Geometry: final body of the model. Coordinates: model frame, mm. Face numbers are marked on the shaded views. A direction names the side the tool comes from. Give positions to 0.01 mm unless a question says otherwise; leave off trailing zeros. Write each loop counter-clockwise with the first axis right and the second up, starting at its lowest first coordinate (ties: lowest second). Pieces come first, ordered by that corner, then holes.
Q1. Section B-B (x = 10). Return the cut outline in (y, z).
Q2. Section D-D (z = -4.25). Return the cut outline in (x, y).
Q3. Section C-C (x = -4). Return the cut outline in (y, z), plus the area to 3 significant figures.
Q4. Line query: line 1 (X direction, y = 8, z = -7); line 2 (X direction, y = 15.5, z = -4); line 3 (X direction, y = 14.5, z = -2.5). Output: solid intervals per line, ascending.
Q5. Pin query (flat end, axial travel): pin 1 Ø3 at (x, z) = (0, -7) entering from +Y; pin 2 Ø1.5 at (x, z) = (-2.5, -4) entering from +Y. Return the tip coordinate at first contact, or that it passes through.
Q6. Section A-A (y = 9.25). Return the cut outline in (x, z).
Q7. Mould query, pull axis X, two halves, no side actions, for the marked faces 3, 4 and 5. Classes: +X half, -X half, draft (parallel to the pull), parting line (faces both ways), or undercut.
Q8. Reachability of the marked faces 1 and 2 from +Z, -Z, +X, -X, +Y, -Y: full face, straight path, thin tool, end or side. Return the list, or none.
from build123d import *

# Parameters (mm, degrees)
BOSS_EXTRUDE1_DEPTH = 20
BOSS_EXTRUDE2_DEPTH = 16


with BuildPart() as part:
    # Sketch1 → Boss-Extrude1 (new body)
    with BuildSketch(Plane(origin=(0, 0, 0), x_dir=(1, 0, 0), z_dir=(0, 1, 0))):
        with BuildLine():
            Line((-15, 0), (-8, 0))
            Line((-8, 0), (-8, 0.4))
            Line((-8, 0.4), (-12, 4.6))
            Line((-12, 4.6), (-12, 5))
            Line((-12, 5), (-7, 5))
            ThreePointArc((-7, 5), (-5.585786438, 5.585786438), (-5, 7))
            ThreePointArc((-5, 7), (0, 12), (5, 7))
            ThreePointArc((5, 7), (5.585786438, 5.585786438), (7, 5))
            Line((7, 5), (12, 5))
            Line((12, 5), (12, 4.6))
            Line((12, 4.6), (8, 0.4))
            Line((8, 0.4), (8, 0))
            Line((8, 0), (15, 0))
            Line((15, 0), (15, 13))
            Line((15, 13), (-15, 13))
            Line((-15, 13), (-15, 0))
        make_face()
    extrude(amount=BOSS_EXTRUDE1_DEPTH)

    # Sketch1_3 → Boss-Extrude2 (add)
    with BuildSketch(Plane(origin=(0, 0, 0), x_dir=(1, 0, 0), z_dir=(0, 1, 0))):
        with BuildLine():
            ThreePointArc((2, 7), (1.414213562, 5.585786438), (0, 5))
            Line((0, 5), (4.582575695, 5))
            ThreePointArc((4.582575695, 5), (4.894531565, 5.978451782), (5, 7))
            Line((5, 7), (2, 7))
        make_face()
        with BuildLine():
            Line((-4.582575695, 5), (0, 5))
            ThreePointArc((0, 5), (-1.414213562, 8.414213562), (2, 7))
            Line((2, 7), (5, 7))
            ThreePointArc((5, 7), (0, 12), (-5, 7))
            ThreePointArc((-5, 7), (-4.894531565, 5.978451782), (-4.582575695, 5))
        make_face()
        with BuildLine():
            ThreePointArc((-4.582575695, 5), (-2.738612788, 2.816699867), (0, 2))
            Line((0, 2), (0, 5))
            Line((0, 5), (-4.582575695, 5))
        make_face()
        with BuildLine():
            Line((0, 5), (0, 2))
            ThreePointArc((0, 2), (2.738612788, 2.816699867), (4.582575695, 5))
            Line((4.582575695, 5), (0, 5))
        make_face()
        with BuildLine():
            Line((-7, 5), (-4.582575695, 5))
            ThreePointArc((-4.582575695, 5), (-4.894531565, 5.978451782), (-5, 7))
            ThreePointArc((-5, 7), (-5.585786438, 5.585786438), (-7, 5))
        make_face()
        with BuildLine():
            ThreePointArc((5, 7), (4.894531565, 5.978451782), (4.582575695, 5))
            Line((4.582575695, 5), (7, 5))
            ThreePointArc((7, 5), (5.585786438, 5.585786438), (5, 7))
        make_face()
    extrude(amount=BOSS_EXTRUDE2_DEPTH)


solid = part.part
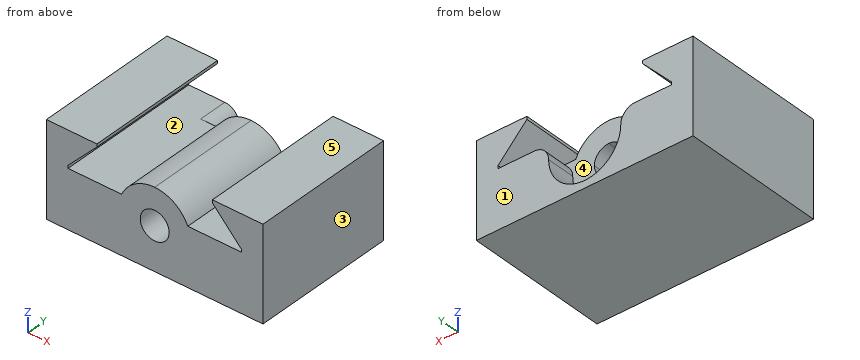
Computed:
1. outline: (0, -13) - (20, -13) - (20, -5) - (0, -5) - close; (0, -2.5) - (20, -2.5) - (20, 0) - (0, 0) - close
2. outline: (-15, 0) - (-11.67, 0) - (-11.67, 20) - (-15, 20) - close; (-4.18, 0) - (4.18, 0) - (4.18, 16) - (-4.18, 16) - close; (11.67, 0) - (15, 0) - (15, 20) - (11.67, 20) - close
3. outline: (0, -13) - (20, -13) - (20, -10) - (16, -10) - (16, -4) - (0, -4) - close
3. area: 156 mm2
4. line 1: x = -15 to -2, 2 to 15
4. line 2: x = -15 to -11.43, -4 to 4, 11.43 to 15
4. line 3: x = -15 to -10, -2.18 to 2.18, 10 to 15
5. pin 1: passes through
5. pin 2: stops at y = 16
6. outline: (-15, -13) - (15, -13) - (15, 0) - (8, 0) - (8, -0.4) - (12, -4.6) - (12, -5) - (4.58, -5) arc R5 ccw to (-4.58, -5) - (-12, -5) - (-12, -4.6) - (-8, -0.4) - (-8, 0) - (-15, 0) - close; hole circle Ø4 at (0, -7)
7. face 3: +X half
7. face 4: undercut
7. face 5: draft
8. face 1: +Z, -Z, +X, -X, +Y
8. face 2: +Y, -Y
